from build123d import *

# Parameters (mm, degrees)
PAD_DEPTH            = 5
SKETCH001_R          = 8
PAD001_DEPTH         = 75
SKETCH002_R          = 12.5
PAD002_DEPTH         = 60
PAD002_TAPER         = 2
SKETCH004_R          = 5
PAD003_DEPTH         = 75
PAD004_DEPTH         = 50
PAD004_TAPER         = 2
FILLET_R             = 4
FILLET001_R          = 1.5
FILLET002_R          = 1
BODY_PLACEMENT_ANGLE = 270


with BuildPart() as part:
    # Sketch → Pad (new body)
    with BuildSketch(Plane.XZ.offset(2.5)):
        Polygon((20, 75), (10, 75), (10, 5), (15, 5), (20, 10), (20, 15), (15, 20), (15, 25), (20, 30), align=None)
    extrude(amount=PAD_DEPTH)

    # Sketch001 → Pad001 (join)
    with BuildSketch(Plane.XY.offset(75)):
        with Locations((10, -5)):
            Circle(SKETCH001_R)
    extrude(amount=PAD001_DEPTH)

    # Sketch002 → Pad002 (join)
    with BuildSketch(Plane.XY.offset(150)):
        with Locations((10, -5)):
            Circle(SKETCH002_R)
    extrude(amount=-PAD002_DEPTH, taper=PAD002_TAPER)

    # Sketch004 → Pad003 (join)
    with BuildSketch(Plane.XY.offset(5)):
        with Locations((10, -5)):
            Circle(SKETCH004_R)
    extrude(amount=PAD003_DEPTH)

    # Sketch003 → Pad004 (join)
    with BuildSketch(Plane.XY.offset(145)):
        Polygon((11.5, -4), (11.5, -6), (23.5, -8), (23.5, -2), align=None)
        Polygon((11, -6.5), (9, -6.5), (7, -18.5), (13, -18.5), align=None)
        Polygon((8.5, -6), (8.5, -4), (-3.5, -2), (-3.5, -8), align=None)
        Polygon((9, -3.5), (11, -3.5), (13, 8.5), (7, 8.5), align=None)
    extrude(amount=-PAD004_DEPTH, taper=PAD004_TAPER)

    # Fillet
    fillet_edges = [part.edges().sort_by_distance(p)[0] for p in [
        (-2.5, -5, 150),
    ]]
    fillet(fillet_edges, radius=FILLET_R)

    # Fillet001
    fillet001_edges = [part.edges().sort_by_distance(p)[0] for p in [
        (-0.404754, -5, 90),
    ]]
    fillet(fillet001_edges, radius=FILLET001_R)

    # Fillet002
    fillet002_edges = [part.edges().sort_by_distance(p)[0] for p in [
        (14.665064, -2.5, 5),
        (15, -5, 5),
        (14.665064, -7.5, 5),
        (5, -5, 5),
        (20, -5, 30),
        (20, -5, 75),
        (20, -2.5, 52.5),
        (20, -7.5, 52.5),
        (20, -5, 15),
        (20, -5, 10),
        (20, -2.5, 12.5),
        (20, -7.5, 12.5),
    ]]
    fillet(fillet002_edges, radius=FILLET002_R)


with BuildPart() as part_1:
    # Body placement: moved
    add(part.part.moved(Location((-5, 25, -45))).rotate(Axis((-5, 25, -45), (0, 0, -1)), BODY_PLACEMENT_ANGLE))


solid = part_1.part
Geometry: final body of the model. Coordinates: model frame, mm. A direction names the side the tool comes from. Round coordinates to 2 decimals unless told otherwise and drop trailing zeros. Order: outer loops, then holes, each group sorted by start corner. A loop starts at its lowest first (then second) coordinate and runs counter-clockwise, first axis right, second up.
Q1. Access query for faces 1 (the face through (-2.5, 42, -4)), 2 (the face through (2.5, 42, -4)), 3 (the face through (0, 45, 7)). Directions: +Z, -Z, +X, -X, +Y, -Y. A direction counts if a zero-diameter tool reaches every point of the face in a straight line with its end or side. Return the directions, or none.
Result sheet:
face 1: -Z, -X, +Y
face 2: -Z, +X, +Y
face 3: -Z, +X, -X, +Y
Q2. Mould query, pull axis Z, two halves, no side actions, for faces 4 (the face through (0, 42, -18)), 5 (the face through (0, 29, 30)), 6 (the face through (0, 35, 105)). Classes: released by +Z, released by -Z, zero draft, split by the parting line, or undercut.
Result sheet:
face 4: undercut
face 5: released by -Z
face 6: released by +Z
Q3. Section B-B, the plane z = 42. Output: boundary loops of the cut face in (x, y), and give its area (3 significant figures).
Result sheet:
outline: circle Ø16 at (0, 35)
area: 201 mm2
Q4. Material intervals for probe 1 along Z at (x, y) = (-0.25, 44.5); probe 2 along Z at (x, y) = (-0.5, 26.5); probe 3 along X at (y, z) = (44, -8), sorted ascending.
Result sheet:
probe 1: z = -35.5 to -29.5, -15.5 to 29.87, 45.1 to 104.83
probe 2: z = 45 to 105
probe 3: x = -2.5 to 2.5
Q5. Section A-A, the plane z = 9. Output: boundary loops of the cut face in (x, y).
Result sheet:
outline: (-2.5, 39.33) arc R5 ccw (long way) to (2.5, 39.33) - (2.5, 44) arc R1 ccw to (1.5, 45) - (-1.5, 45) arc R1 ccw to (-2.5, 44) - close
Q6. Pin query (flat end, axial travel): pin 1 (3 mm diameter, centred on y = 26.5, z = 58.5, fed in from -X); pin 2 (4 mm diameter, centred on y = 41, z = -20, fed in from -X); pin 3 (1.5 mm diameter, centred on x = -0.5, z = 17, fed in from +Y). Return the tip coordinate at first contact, or that it passes through.
Result sheet:
pin 1: stops at x = -8.33
pin 2: stops at x = -3
pin 3: stops at y = 45
